```python
from build123d import *

# Parameters (mm, degrees)
SKETCH3_W          = 30
SKETCH3_H          = 2
CHAMFER1_SIZE      = 0.6
CUT_EXTRUDE1_DEPTH = 1.61
SKETCH9_R          = 1.443375673
CUT_EXTRUDE2_DEPTH = 1.61
CUT_EXTRUDE2_DRAFT = -45


with BuildPart() as part:
    # Sketch3 → Revolve1 (revolve)
    with BuildSketch(Plane(origin=(0, 0, 0), x_dir=(0, 0, -1), z_dir=(1, 0, 0))):
        with Locations((0, 1)):
            Rectangle(SKETCH3_W, SKETCH3_H)
    revolve(axis=Axis((0, 0, -15), (0, 0, 1)))

    # Chamfer1
    chamfer1_edges = [part.edges().sort_by_distance(p)[0] for p in [
        (0, -2, -15),
    ]]
    chamfer(chamfer1_edges, length=CHAMFER1_SIZE)

    # Sketch6 → Revolve2 (revolve)
    with BuildSketch(Plane(origin=(0, 0, 0), x_dir=(0, 0, -1), z_dir=(1, 0, 0))):
        Polygon((-15, 4), (-14.7, 4), (-12.7, 2), (-12.7, 0), (-15, 0), align=None)
    revolve(axis=Axis((0, 0, -15), (0, 0, 1)))

    # Sketch8 → Cut-Extrude1 (cut)
    with BuildSketch(Plane.XY.offset(15)):
        Polygon((0, 1.443375673), (-1.25, 0.721687836), (-1.25, -0.721687836), (0, -1.443375673), (1.25, -0.721687836), (1.25, 0.721687836), align=None)
    extrude(amount=-CUT_EXTRUDE1_DEPTH, mode=Mode.SUBTRACT)


with BuildPart() as cut_extrude2_tool:
    # Sketch9 → Cut-Extrude2 (with draft: the straight prism first)
    with BuildSketch(Plane.XY.offset(15)):
        Circle(SKETCH9_R)
    extrude(amount=-CUT_EXTRUDE2_DEPTH)
    # Cut-Extrude2: the draft: its side faces are tilted about the plane it starts from
    cut_extrude2_sides = [cut_extrude2_tool.faces().sort_by_distance(p)[0] for p in [
        (-1.443375673, 0, 14.195),
    ]]
    draft(cut_extrude2_sides, Plane.XY.offset(15), CUT_EXTRUDE2_DRAFT)


with BuildPart() as part_1:
    add(part.part)

    # Cut-Extrude2: cut by cut_extrude2_tool
    add(cut_extrude2_tool.part, mode=Mode.SUBTRACT)


solid = part_1.part
```
Geometry: final body of the model. Coordinates: model frame, mm. A direction names the side the tool comes from. Coordinates: 2 decimals unless noted, no trailing zeros. Loops run counter-clockwise (first coordinate to the right, second up) from the corner with the lowest first, then second, coordinate; pieces in that order, holes last. Notation, with made-up numbers: (23.25, 52.5) -> (65.25, 52.5) arc R26 ccw to (65.25, 78.5) -> close; hole circle Ø9 at (10.5, -1.5). An arc over 180 degrees is marked (long way). Use a Markdown table: item, result. Add a question column.
(1) Pin query (flat end, axial travel): pin 1 Ø1 at (x, y) = (-1.5, 3) entering from -Z; pin 2 Ø4 at (y, z) = (-2, 6) entering from +X; pin 3 Ø0.7 at (y, z) = (0, 14) entering from -X. Return the tip coordinate at first contact, or that it passes through.
(2) Mould query, pull axis Y, two halves, no side actions, for faces 1 (the flat face through (0, 0, -15)), 2 (the flat face through (-0.63, -1.08, 14.21)), 3 (the cylindrical face through (2, 0, -1)). Classes: pulls with the +Y half, pulls with the -Y half, needs draft (parallel to the pull), parting line crosses it, or undercut.
(3) Section query B-B, the plane z = -2.25. Return loops of the section in (x, y), plus the area to 3 significant figures.
(4) Line query: line 1 along Z through (x, y) = (0, 0); line 2 along X through (y, z) = (0, 3.5); line 3 along Z through (x, y) = (0.5, 2.5). Output: solid intervals per line, ascending.
(5) Access query for faces 4 (the flat face through (0, 0, 13.39)), 5 (the flat face through (0, -2, 15)). Directions: +Z, -Z, +X, -X, +Y, -Y. A direction counts if a zero-diameter tool reaches every point of the face in a straight line with its end or side. Return the directions, or none.
(6) Section query A-A, the plane y = 0. Return loops of the section in (x, z), plus the area to 3 significant figures.
Answer:
| question | item | result |
|---|---|---|
| 1 | pin 1 | stops at z = 13.55 |
| 1 | pin 2 | stops at x = 2 |
| 1 | pin 3 | stops at x = -3.65 |
| 2 | face 1 | needs draft |
| 2 | face 2 | undercut |
| 2 | face 3 | parting line crosses it |
| 3 | outline | circle Ø4 at (0, 0) |
| 3 | area | 12.6 mm^2 |
| 4 | line 1 | z = -15 to 13.39 |
| 4 | line 2 | x = -2 to 2 |
| 4 | line 3 | z = 13.25 to 15 |
| 5 | face 4 | +Z |
| 5 | face 5 | +Z, +X, -X, +Y, -Y |
| 6 | outline | (-4, 14.7) -> (-2, 12.7) -> (-2, -14.4) -> (-1.4, -15) -> (1.4, -15) -> (2, -14.4) -> (2, 12.7) -> (4, 14.7) -> (4, 15) -> (1.44, 15) -> (1.25, 14.81) -> (1.25, 13.39) -> (-1.25, 13.39) -> (-1.25, 14.81) -> (-1.44, 15) -> (-4, 15) -> close |
| 6 | area | 121 mm^2 |
